from build123d import *

# Parameters (mm, degrees)
F0_R     = 40.160113
F1_DEPTH = 60.96
F3_DEPTH = 183.896


with BuildPart() as f1:
    # F0 (on Top) → F1 (new body)
    with BuildSketch(Plane.XY):
        Circle(F0_R)
    extrude(amount=F1_DEPTH)

    # F2 (on face) → F3 (cut)
    with BuildSketch(Plane.XY.offset(60.96)):
        Polygon((-12.354089, -29.82541), (12.354089, -29.82541), (29.82541, -12.354089), (29.82541, 12.354089), (12.354089, 29.82541), (-12.354089, 29.82541), (-29.82541, 12.354089), (-29.82541, -12.354089), align=None)
    extrude(amount=-F3_DEPTH, mode=Mode.SUBTRACT)


solid = f1.part
Geometry: final body of the model. Coordinates: model frame, mm. A direction names the side the tool comes from. Round coordinates to 2 decimals unless told otherwise and drop trailing zeros. Loops run counter-clockwise (first coordinate to the right, second up) from the corner with the lowest first, then second, coordinate; pieces in that order, holes last.
Q1. Pull-direction query (Y, two-part tool) for faces 3 (the flat face through (-3, 30, 60.96)), 4 (the flat face through (-20.97, 21.21, 30.91)), 5 (the cylindrical face through (38.306, 12.063, 30.053)); classes: released by +Y, released by -Y, zero draft, split by the parting line, or undercut.
Q2. Material intervals for L1, parallel to X at y = 23, z = 29.5; L2, parallel to Y at x = -8, z = 47; L3, parallel to X at y = 3.5, z = 6.5, sorted ascending.
Q3. Access query for faces 1 (the flat face through (21.21, 20.97, 30.91)), 2 (the flat face through (-3, 30, 0)). Directions: +Z, -Z, +X, -X, +Y, -Y. A direction counts if a zero-diameter tool reaches every point of the face in a straight line with its end or side. Return the directions, or none.
Q4. Section A-A on y = 0. Return loops of the section in (x, z).
Q5. Pin query (flat end, axial travel): P1, Ø8, axis at x = 2, z = 44, coming from the -Y side; P2, Ø1.5, axis at y = -19, z = 20, coming from the +X side; P3, Ø2, axis at y = 15.5, z = 22, coming from the -X side. Return the tip coordinate at first contact, or that it passes through.
Q6. Section D-D on x = -32.5. Return loops of the section in (y, z), plus the area to 3 significant figures.
Q7. Section C-C on z = 29.5. Return loops of the section in (x, y), plus the area to 3 significant figures.
Evaluation:
1. face 3: zero draft
1. face 4: undercut
1. face 5: split by the parting line
2. L1: x = -32.92 to -19.18, 19.18 to 32.92
2. L2: y = -39.36 to -29.83, 29.83 to 39.36
2. L3: x = -40.01 to -29.83, 29.83 to 40.01
3. face 1: +Z, -Z
3. face 2: -Z, +X, -X, +Y, -Y
4. outline: (-40.16, 0) - (-29.83, 0) - (-29.83, 60.96) - (-40.16, 60.96) - close; (29.83, 0) - (40.16, 0) - (40.16, 60.96) - (29.83, 60.96) - close
5. P1: stops at y = -40.16
5. P2: stops at x = 35.77
5. P3: stops at x = -37.45
6. outline: (-23.59, 0) - (23.59, 0) - (23.59, 60.96) - (-23.59, 60.96) - close
6. area: 2,880 mm2
7. outline: circle Ø80.32 at (0, 0); hole (-29.83, -12.35) - (-12.35, -29.83) - (12.35, -29.83) - (29.83, -12.35) - (29.83, 12.35) - (12.35, 29.83) - (-12.35, 29.83) - (-29.83, 12.35) - close
7. area: 2,120 mm2
